```python
from build123d import *

# Parameters (mm, degrees)
PAD_DEPTH    = 15
CHAMFER_SIZE = 0.4


with BuildPart() as part:
    # Sketch → Pad (new body)
    with BuildSketch(Plane.XY):
        with BuildLine():
            ThreePointArc((-17.5, 19.1), (-36.6, 0), (-17.5, -19.1))
            Line((-17.5, -19.1), (17.5, -19.1))
            ThreePointArc((17.5, -19.1), (36.6, 0), (17.5, 19.1))
            Line((-17.5, 19.1), (17.5, 19.1))
        make_face()
        with BuildLine():
            ThreePointArc((-17.5, 17.5), (-35, 0), (-17.5, -17.5))
            Line((-17.5, -17.5), (17.5, -17.5))
            ThreePointArc((17.5, -17.5), (35, 0), (17.5, 17.5))
            Line((-17.5, 17.5), (17.5, 17.5))
        make_face(mode=Mode.SUBTRACT)
    extrude(amount=PAD_DEPTH)

    # Chamfer
    chamfer_edges = [part.edges().sort_by_distance(p)[0] for p in [
        (-36.6, 0, 15),
        (0, -19.1, 15),
        (36.6, 0, 15),
        (0, 19.1, 15),
        (-35, 0, 15),
        (0, -17.5, 15),
        (35, 0, 15),
        (0, 17.5, 15),
        (-36.6, 0, 0),
        (0, -19.1, 0),
        (36.6, 0, 0),
        (0, 19.1, 0),
        (-35, 0, 0),
        (0, -17.5, 0),
        (35, 0, 0),
        (0, 17.5, 0),
    ]]
    chamfer(chamfer_edges, length=CHAMFER_SIZE)


solid = part.part
```
Part model, mm, in its own coordinate system. A direction names the side the tool comes from. Round coordinates to 2 decimals unless told otherwise and drop trailing zeros. Loops run counter-clockwise (first coordinate to the right, second up) from the corner with the lowest first, then second, coordinate; pieces in that order, holes last.
1. Drill centre lines: line 1 along Y through (x, z) = (-15, 3.5); line 2 along X through (y, z) = (0.5, 14); line 3 along Y through (x, z) = (21, 9.75). Where is each one in solid material? Low to high.
Solutions:
line 1: y = -19.1 to -17.5, 17.5 to 19.1
line 2: x = -36.59 to -34.99, 34.99 to 36.59
line 3: y = -18.78 to -17.15, 17.15 to 18.78
2. Flat gauge pins, fed straight in: pin 1 (1.5 mm diameter, centred on y = -6.5, z = 11, fed in from +X); pin 2 (3 mm diameter, centred on x = 20.5, z = 11.5, fed in from +Y); pin 3 (1 mm diameter, centred on y = -12, z = 12, fed in from -X). Where does each tip first touch, or does it go through?
Solutions:
pin 1: stops at x = 35.71
pin 2: stops at y = 19.04
pin 3: stops at x = -32.75
3. Two-plate mould, pull along Y, no slides. Class faces 5 (the face through (35, 0, 7)), 6 (the face through (-35, 0, 7)), 7 (the face through (36.595, -0.42, 7.401)), 8 (the face through (-0.2, 18.1, 0)): pulls with the +Y half, pulls with the -Y half, needs draft (parallel to the pull), parting line crosses it, or undercut.
Solutions:
face 5: undercut
face 6: undercut
face 7: parting line crosses it
face 8: needs draft
4. Slice it at B-B (y = 0). Give the cut face in (x, z).
Solutions:
outline: (-36.6, 0.4) - (-36.2, 0) - (-35.4, 0) - (-35, 0.4) - (-35, 14.6) - (-35.4, 15) - (-36.2, 15) - (-36.6, 14.6) - close; (35, 0.4) - (35.4, 0) - (36.2, 0) - (36.6, 0.4) - (36.6, 14.6) - (36.2, 15) - (35.4, 15) - (35, 14.6) - close
5. Slice it at A-A (z = 11). Give the cut face in (x, y).
Solutions:
outline: (-17.5, -19.1) - (17.5, -19.1) arc R19.1 ccw to (17.5, 19.1) - (-17.5, 19.1) arc R19.1 ccw to start; hole (-17.5, -17.5) - (17.5, -17.5) arc R17.5 ccw to (17.5, 17.5) - (-17.5, 17.5) arc R17.5 ccw to start
6. 3-axis set-ups, long thin cutter, end or side, ignore diameter. For faces 1 (the face through (0, 17.5, 7)), 2 (the face through (-35.11, 0.387, 0.286)), 3 (the face through (35.11, -0.387, 14.714)), 4 (the face through (0, 19.1, 7)): which of +Z, -Z, +X, -X, +Y, -Y reach the whole face in a straight line?
Solutions:
face 1: +Z, -Z
face 2: -Z
face 3: +Z
face 4: +Z, -Z, +X, -X, +Y
